Verification items for this drawing (mm, ordinates from the low corner). A direction names the side the tool comes from. Give positions to 0.01 mm unless a question says otherwise; leave off trailing zeros. Loops run counter-clockwise (first coordinate to the right, second up) from the corner with the lowest first, then second, coordinate; pieces in that order, holes last. Notation, with made-up numbers: (-22.5, 47) -> (33.5, 47) arc R11 cw to (33.5, 67) -> close; hole circle Ø5 at (34, -38.75). An arc over 180 degrees is marked (long way). Answer in a Markdown table with one row per item. Add a question column.
Q1. Section check C-C on y = 9.25. Enter the section's corners in (x, z).
Q2. Section check A-A on x = 17.5. Enter the section's corners in (y, z).
Q3. Section check D-D on z = 10. Enter the section's corners in (x, y).
Q4. Gauge pin test, flat ends, axial feed: P1, Ø3, axis at x = 26.5, y = 10, coming from the +Z side; P2, Ø5, axis at x = 6.5, z = 5, coming from the +Y side; P3, Ø4, axis at y = 5, z = 27, coming from the -X side. Record the tip position at first contact, or that the pin passes through.
Q5. Material ranges on probe 1 along Z at (x, y) = (17.5, 1.8); probe 2 along Y at (x, z) = (10.5, 17.5); probe 3 along X at (y, z) = (7, 17.5), recorded low to high.
Q6. Section check B-B on z = 17.5. Enter the section's corners in (x, y), and give its area (3 significant figures).
Q7. Release check for a two-part mould opening along X. For the marked faces 1, 2 and 3 record: pulls with the +X half, pulls with the -X half, needs draft (parallel to the pull), parting line crosses it, or undercut.
Q8. Set-up check for the marked faces 4 and 5: record each of +Z, -Z, +X, -X, +Y, -Y from which the full face is reachable in a straight line by a thin tool's end or side.
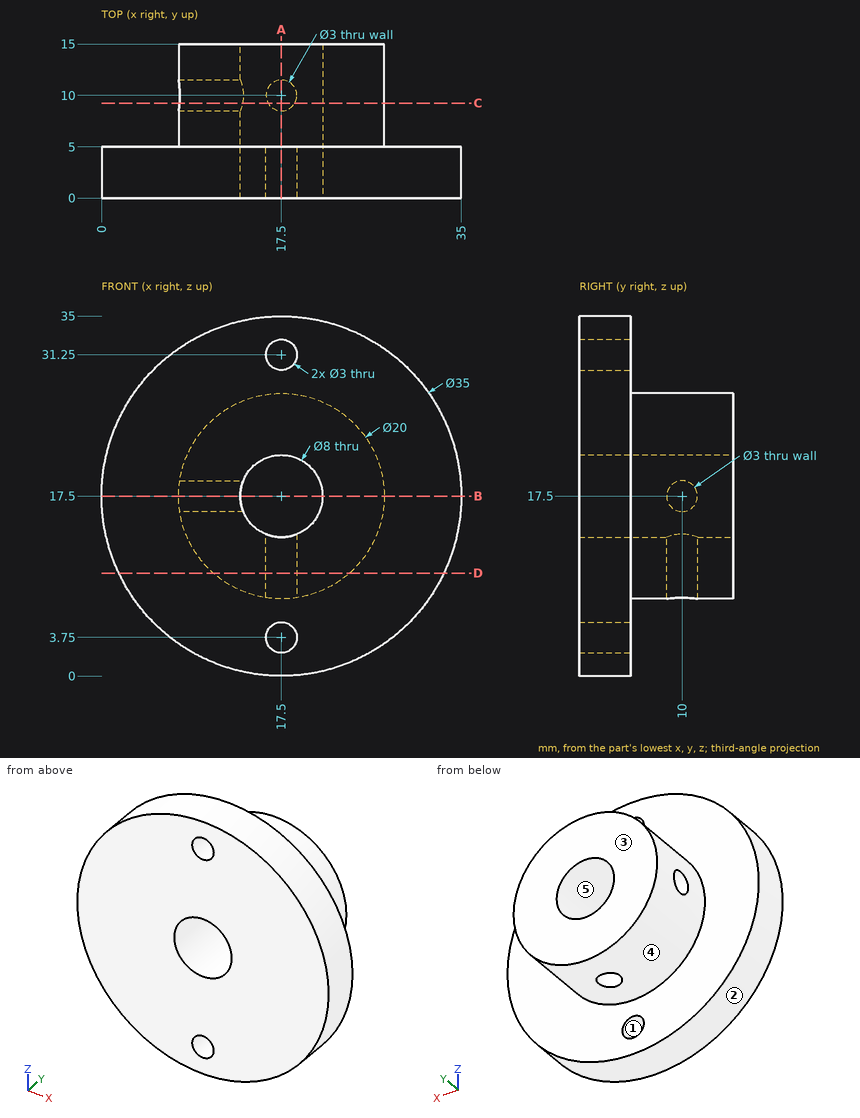
Taken from the geometry:
| question | item | result |
|---|---|---|
| 1 | outline | (7.58, 16.2) arc R10 ccw to (16.2, 7.58) -> (16.2, 13.72) arc R4 cw to (13.72, 16.2) -> close; (7.58, 18.8) -> (13.72, 18.8) arc R4 cw (long way) to (18.8, 13.72) -> (18.8, 7.58) arc R10 ccw (long way) to start |
| 2 | outline | (0, 0) -> (5, 0) -> (5, 2.25) -> (0, 2.25) -> close; (0, 5.25) -> (5, 5.25) -> (5, 7.5) -> (8.5, 7.5) -> (8.5, 13.5) -> (0, 13.5) -> close; (0, 21.5) -> (15, 21.5) -> (15, 27.5) -> (5, 27.5) -> (5, 29.75) -> (0, 29.75) -> close; (0, 32.75) -> (5, 32.75) -> (5, 35) -> (0, 35) -> close; (11.5, 7.5) -> (15, 7.5) -> (15, 13.5) -> (11.5, 13.5) -> close |
| 3 | outline | (1.69, 0) -> (33.31, 0) -> (33.31, 5) -> (24.11, 5) -> (24.11, 15) -> (10.89, 15) -> (10.89, 5) -> (1.69, 5) -> close; hole circle Ø3 at (17.5, 10) |
| 4 | P1 | stops at z = 24.11 |
| 4 | P2 | stops at y = 5 |
| 4 | P3 | stops at x = 1.69 |
| 5 | probe 1 | z = 0 to 2.25, 5.25 to 13.5, 21.5 to 29.75, 32.75 to 35 |
| 5 | probe 2 | y = 0 to 8.5, 11.5 to 15 |
| 5 | probe 3 | x = 7.5 to 13.5, 21.5 to 27.5 |
| 6 | outline | (0, 0) -> (13.5, 0) -> (13.5, 8.5) -> (7.5, 8.5) -> (7.5, 5) -> (0, 5) -> close; (7.5, 11.5) -> (13.5, 11.5) -> (13.5, 15) -> (7.5, 15) -> close; (21.5, 0) -> (35, 0) -> (35, 5) -> (27.5, 5) -> (27.5, 15) -> (21.5, 15) -> close |
| 6 | area | 237 mm² |
| 7 | face 1 | undercut |
| 7 | face 2 | parting line crosses it |
| 7 | face 3 | needs draft |
| 8 | face 4 | +Y |
| 8 | face 5 | +Y, -Y |
